Check sheet for the modelled part. Datum: model origin and axes. Units: mm. Round coordinates to 2 decimals unless told otherwise and drop trailing zeros. Order: outer loops, then holes, each group sorted by start corner. A loop starts at its lowest first (then second) coordinate and runs counter-clockwise, first axis right, second up.
from build123d import *

# Parameters (mm, degrees)
PAD_DEPTH       = 232
POCKET_DEPTH    = 10
POCKET001_DEPTH = 10
SKETCH003_W     = 3.95
SKETCH003_H     = 16
POCKET002_DEPTH = 10


with BuildPart() as part:
    # Sketch → Pad (new body)
    with BuildSketch(Plane.XY):
        with BuildLine():
            ThreePointArc((0, 36.7), (-25.9508188695, 25.9508188695), (-36.7, 0))
            Line((-39.7, 0), (-36.7, 0))
            ThreePointArc((0, 39.7), (-28.0721392131, 28.0721392131), (-39.7, 0))
            Line((0, 36.7), (0, 39.7))
        make_face()
    extrude(amount=PAD_DEPTH)

    # Sketch001 (on Face6 of Pad) → Pocket (cut)
    with BuildSketch(Plane.XY.offset(232)):
        with BuildLine():
            Line((-34.546220009, 12.3874405384), (-37.3653275389, 13.4135117665))
            ThreePointArc((-34.3734039674, 19.8635117665), (-36.0140531533, 16.70562706), (-37.3653275389, 13.4135117665))
            Line((-34.3734039674, 19.8635117665), (-31.7753275389, 18.3635116412))
            ThreePointArc((-31.7753275389, 18.3635116412), (-33.2951238734, 15.4377694716), (-34.546220009, 12.3874405384))
        make_face()
        with BuildLine():
            ThreePointArc((-12.5518984396, 34.4868068334), (-15.5057350305, 33.2635262888), (-18.3418983946, 31.7878084064))
            Line((-18.3418983946, 31.7878084064), (-19.8418984396, 34.3858846958))
            ThreePointArc((-13.5779588696, 37.3058846958), (-16.7735898258, 35.9824496714), (-19.8418984396, 34.3858846958))
            Line((-13.5779588696, 37.3058846958), (-12.5518984396, 34.4868068334))
        make_face()
    extrude(amount=-POCKET_DEPTH, mode=Mode.SUBTRACT)

    # Sketch002 (on Face5 of Pad) → Pocket001 (cut)
    with BuildSketch(Plane(origin=(0, 0, 0), x_dir=(1, 0, 0), z_dir=(0, 0, -1))):
        with BuildLine():
            ThreePointArc((-37.3090779514, -13.5691820834), (-35.9850847763, -16.767935879), (-34.3874519885, -19.8391820834))
            Line((-31.789375638, -18.3391820031), (-34.3874519885, -19.8391820834))
            ThreePointArc((-34.49, -12.543121621), (-33.2661613014, -15.5000810407), (-31.789375638, -18.3391820031))
            Line((-34.49, -12.543121621), (-37.3090779514, -13.5691820834))
        make_face()
        with BuildLine():
            Line((-12.5521392601, -34.4867191828), (-13.57819969, -37.3057970452))
            ThreePointArc((-19.8453837991, -34.3838732819), (-16.7755295873, -35.981545368), (-13.57819969, -37.3057970452))
            Line((-18.3453837845, -31.7857970452), (-19.8453837991, -34.3838732819))
            ThreePointArc((-18.3453837845, -31.7857970452), (-15.507674799, -33.2626220002), (-12.5521392601, -34.4867191828))
        make_face()
    extrude(amount=-POCKET001_DEPTH, mode=Mode.SUBTRACT)

    # Sketch003 (on Face14 of Pocket001) → Pocket002 (cut)
    with BuildSketch(Plane.XZ):
        with Locations((-38.245, 121)):
            Rectangle(SKETCH003_W, SKETCH003_H)
    extrude(amount=-POCKET002_DEPTH, mode=Mode.SUBTRACT)


solid = part.part
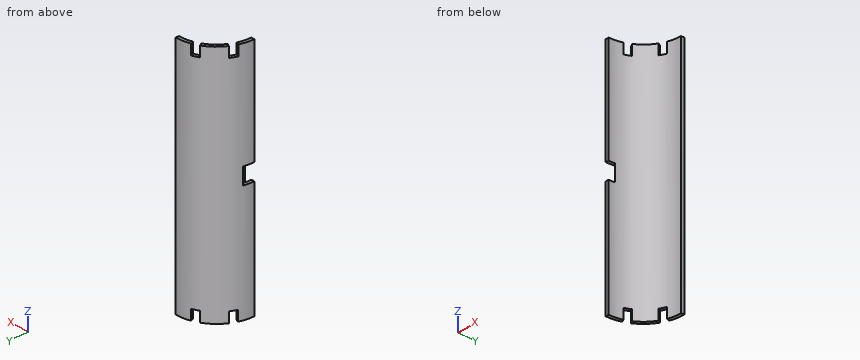
1) Sectioned sample at A-A on z = 115. Record the cut outline in (x, y).
2) Gauge pin test, flat ends, axial feed: pin 1 (3 mm diameter, centred on y = 7.5, z = 190.5, fed in from +X); pin 2 (6 mm diameter, centred on x = -20, z = 112.5, fed in from -Y); pin 3 (6 mm diameter, centred on x = -19.5, z = 99.5, fed in from -Y); pin 4 (4 mm diameter, centred on x = -38.5, y = 6, fed in from -Z). Record the tip position at first contact, or that the pin passes through.
3) Sectioned sample at B-B on y = 24. Record the cut outline in (x, z).
4) Scan lines: line 1 (X direction, y = 6.5, z = 109); line 2 (Y direction, x = -5, z = 54); line 3 (X direction, y = 31.5, z = 217). Record each from-to range of solid material in increasing order.
5) Sectioned sample at C-C on x = -27. Record the cut outline in (y, z), and give its area (3 significant figures).
Values found:
1. outline: (-38.42, 10) - (-36.27, 10) - (-36.27, 5.6) arc R36.7 cw to (0, 36.7) - (0, 39.7) arc R39.7 ccw to start
2. pin 1: stops at x = -35.58
2. pin 2: stops at y = 28.6
2. pin 3: stops at y = 28.99
2. pin 4: stops at z = 0
3. outline: (-31.62, 0) - (-27.76, 0) - (-27.76, 232) - (-31.62, 232) - close
4. line 1: x = -39.16 to -36.12
4. line 2: y = 36.36 to 39.38
4. line 3: x = -24.16 to -18.83
5. outline: (24.86, 0) - (29.1, 0) - (29.1, 232) - (24.86, 232) - close
5. area: 985 mm2
